from build123d import *

# Parameters (mm, degrees)
SKETCH_1_R      = 1.6
SKETCH_1_R_2    = 1.1
EXTRUDE_1_DEPTH = 5
SKETCH_2_R      = 1.6
SKETCH_2_R_2    = 1.1
EXTRUDE_2_DEPTH = 4
EXTRUDE_START   = 4
SKETCH_3_R      = 1.1
SKETCH_3_R_2    = 1.3
EXTRUDE_3_DEPTH = 4
FILLET_2_R      = 2.5
SKETCH_4_W      = 16
SKETCH_4_H      = 46
EXTRUDE_4_DEPTH = 4
FILLET_3_R      = 5


with BuildPart() as part:
    # Sketch 1 → Extrude 1 (new body)
    with BuildSketch(Plane.XY):
        with BuildLine():
            Line((-8, 0), (8, 0))
            Line((8, 0), (8, 12))
            ThreePointArc((8, 12), (10, 18), (8, 24))
            Line((8, 24), (8, 36))
            Line((8, 36), (-8, 36))
            Line((-8, 36), (-8, 24))
            ThreePointArc((-8, 24), (-10, 18), (-8, 12))
            Line((-8, 12), (-8, 0))
        make_face()
        with Locations((0, 18)):
            Circle(SKETCH_1_R, mode=Mode.SUBTRACT)
        with Locations((0, 24)):
            Circle(SKETCH_1_R_2, mode=Mode.SUBTRACT)
        with Locations((4.242640687, 22.242640687)):
            Circle(SKETCH_1_R_2, mode=Mode.SUBTRACT)
        with Locations((6, 18)):
            Circle(SKETCH_1_R_2, mode=Mode.SUBTRACT)
        with Locations((4.242640687, 13.757359313)):
            Circle(SKETCH_1_R_2, mode=Mode.SUBTRACT)
        with Locations((0, 12)):
            Circle(SKETCH_1_R_2, mode=Mode.SUBTRACT)
        with Locations((-4.242640687, 13.757359313)):
            Circle(SKETCH_1_R_2, mode=Mode.SUBTRACT)
        with Locations((-6, 18)):
            Circle(SKETCH_1_R_2, mode=Mode.SUBTRACT)
        with Locations((-4.242640687, 22.242640687)):
            Circle(SKETCH_1_R_2, mode=Mode.SUBTRACT)
    extrude(amount=EXTRUDE_1_DEPTH)

    # Sketch 2 → Extrude 2 (add)
    with BuildSketch(Plane.XZ):
        with BuildLine():
            Line((-8, 0), (8, 0))
            Line((8, 0), (8, 21))
            ThreePointArc((8, 21), (10, 27), (8, 33))
            Line((8, 33), (8, 37))
            Line((8, 37), (-8, 37))
            Line((-8, 37), (-8, 33))
            ThreePointArc((-8, 33), (-10, 27), (-8, 21))
            Line((-8, 21), (-8, 0))
        make_face()
        with Locations(Location((0, 27, 0), (0, 0, 270))):
            Circle(SKETCH_2_R, mode=Mode.SUBTRACT)
        with Locations(Location((6, 27, 0), (0, 0, 270))):
            Circle(SKETCH_2_R_2, mode=Mode.SUBTRACT)
        with Locations(Location((4.242640687, 22.757359313, 0), (0, 0, 270))):
            Circle(SKETCH_2_R_2, mode=Mode.SUBTRACT)
        with Locations(Location((0, 21, 0), (0, 0, 270))):
            Circle(SKETCH_2_R_2, mode=Mode.SUBTRACT)
        with Locations(Location((-4.242640687, 22.757359313, 0), (0, 0, 270))):
            Circle(SKETCH_2_R_2, mode=Mode.SUBTRACT)
        with Locations(Location((-6, 27, 0), (0, 0, 270))):
            Circle(SKETCH_2_R_2, mode=Mode.SUBTRACT)
        with Locations(Location((-4.242640687, 31.242640687, 0), (0, 0, 270))):
            Circle(SKETCH_2_R_2, mode=Mode.SUBTRACT)
        with Locations(Location((0, 33, 0), (0, 0, 270))):
            Circle(SKETCH_2_R_2, mode=Mode.SUBTRACT)
        with Locations(Location((4.242640687, 31.242640687, 0), (0, 0, 270))):
            Circle(SKETCH_2_R_2, mode=Mode.SUBTRACT)
    extrude(amount=EXTRUDE_2_DEPTH)

    # Sketch 3 → Extrude 3 (add)
    with BuildSketch(Plane(origin=(0, 36, 0), x_dir=(1, 0, 0), z_dir=(0, 1, 0)).offset(EXTRUDE_START)):
        with BuildLine():
            Line((8, -5), (8, 0))
            Line((8, 0), (-8, 0))
            Line((-8, 0), (-8, -5))
            Line((-8, -5), (-8, -21))
            ThreePointArc((-8, -21), (-10, -27), (-8, -33))
            Line((-8, -33), (-8, -37))
            Line((-8, -37), (8, -37))
            Line((8, -37), (8, -33))
            ThreePointArc((8, -33), (10, -27), (8, -21))
            Line((8, -21), (8, -5))
        make_face()
        with Locations(Location((4.242640687, -22.757359313, 0), (0, 0, 90))):
            Circle(SKETCH_3_R, mode=Mode.SUBTRACT)
        with Locations(Location((0, -21, 0), (0, 0, 90))):
            Circle(SKETCH_3_R, mode=Mode.SUBTRACT)
        with Locations(Location((-4.242640687, -22.757359313, 0), (0, 0, 90))):
            Circle(SKETCH_3_R, mode=Mode.SUBTRACT)
        with Locations(Location((-6, -27, 0), (0, 0, 90))):
            Circle(SKETCH_3_R, mode=Mode.SUBTRACT)
        with Locations(Location((-4.242640687, -31.242640687, 0), (0, 0, 90))):
            Circle(SKETCH_3_R, mode=Mode.SUBTRACT)
        with Locations(Location((0, -33, 0), (0, 0, 90))):
            Circle(SKETCH_3_R, mode=Mode.SUBTRACT)
        with Locations(Location((4.242640687, -31.242640687, 0), (0, 0, 90))):
            Circle(SKETCH_3_R, mode=Mode.SUBTRACT)
        with Locations(Location((6, -27, 0), (0, 0, 90))):
            Circle(SKETCH_3_R, mode=Mode.SUBTRACT)
        with Locations(Location((0, -27, 0), (0, 0, 270))):
            Circle(SKETCH_3_R_2, mode=Mode.SUBTRACT)
    extrude(amount=-EXTRUDE_3_DEPTH)

    # Fillet 2
    fillet_2_edges = [part.edges().sort_by_distance(p)[0] for p in [
        (8, 38, 21),
        (-8, 38, 21),
        (-8, 38, 33),
        (-8, 38, 37),
        (8, 38, 37),
        (8, 38, 33),
        (-8, 12, 2.5),
        (-8, 24, 2.5),
        (8, 24, 2.5),
        (8, 12, 2.5),
        (-8, -2, 21),
        (8, -2, 21),
        (8, -2, 33),
        (8, -2, 37),
        (-8, -2, 37),
        (-8, -2, 33),
    ]]
    fillet(fillet_2_edges, radius=FILLET_2_R)


with BuildPart() as body_2:
    # Mirror 2: mirrored copy
    add(part.part.mirror(Plane.XY.offset(-18)))


with BuildPart() as part_1:
    add(part.part)

    add(body_2.part)  # Extrude 4 merges body 2
    # Sketch 4 → Extrude 4 (add)
    with BuildSketch(Plane(origin=(0, 40, 0), x_dir=(1, 0, 0), z_dir=(0, 1, 0))):
        with Locations((0, 18)):
            Rectangle(SKETCH_4_W, SKETCH_4_H)
    extrude(amount=-EXTRUDE_4_DEPTH)

    # Fillet 3
    fillet_3_edges = [part_1.edges().sort_by_distance(p)[0] for p in [
        (0, 36, 5),
        (0, 36, 0),
        (0, 36, -36),
        (0, -4, -36),
        (0, 0, -41),
        (0, 36, -41),
        (0, -4, 0),
        (0, 0, 5),
    ]]
    fillet(fillet_3_edges, radius=FILLET_3_R)


solid = part_1.part
Design review of the part built by this model. Coordinates are the model's own, in mm. A direction names the side the tool comes from. Round coordinates to 2 decimals unless told otherwise and drop trailing zeros. Loops run counter-clockwise (first coordinate to the right, second up) from the corner with the lowest first, then second, coordinate; pieces in that order, holes last. Notation, with made-up numbers: M -26,41 L -21,41 A27 ccw -21,64 Z; hole C -13.5,25 d11. An arc over 180 degrees is marked long. Answer as a JSON object with one key per item and string values.
Item 1: Clearance check with flat-ended pins moving along their axes: P1, Ø6, axis at x = -5, y = 21.5, coming from the -Z side; P2, Ø3.5, axis at x = -6, z = 27, coming from the +Y side; P3, Ø16.5, axis at y = 34.5, z = -32.5, coming from the -X side; P4, Ø3.5, axis at x = 6, y = 18, coming from the +Z side. State where each tip first meets the part, or that it passes through.
Answer sheet:
{"P1": "stops at z = -41", "P2": "stops at y = 40", "P3": "stops at x = -8", "P4": "stops at z = 5"}
Item 2: Machinability: for faces 1 (the flat face through (0, 36, -18)), 2 (the flat face through (0, 0, 24)), 3 (the flat face through (2, 18, -41)), which of the approach directions +Z, -Z, +X, -X, +Y, -Y give a long, thin tool a straight path to every point of the face, cutting with its end or side? Answer none if there is none.
Answer sheet:
{"face 1": "+X, -X, -Y", "face 2": "+Z, +X, -X", "face 3": "-Z, +X, -X"}
Item 3: Wall thickness on L1, parallel to X at y = 38, z = 27; L2, parallel to Y at x = -4.5, z = 18.5; L3, parallel to Z at x = -7, y = 30: over which ranges is each line inside the solid? List them lowest first. Write a range as from..to.
Answer sheet:
{"L1": "x = -10..-7.1, -4.9..-1.3, 1.3..4.9, 7.1..10", "L2": "y = -4..0, 36..40", "L3": "z = -41..-36, 0..5"}
Item 4: We need section A-A on y = 18. State how many separate pieces and enclosed holes the cut face has, and give its area (3 significant figures).
Answer sheet:
{"separate pieces": "8", "enclosed holes": "0", "area": "124 mm^2"}
Item 5: The part is to be moulded in two halves that separate along Y. For faces 4 (the cylindrical face through (0.481, -1.972, -61.474)), 5 (the cylindrical face through (0, -2, -37)), 6 (the cylindrical face through (-0.208, 19.586, 2.465)), say which applies: pulls with the +Y half, pulls with the -Y half, needs draft (parallel to the pull), parting line crosses it, or undercut.
Answer sheet:
{"face 4": "needs draft", "face 5": "pulls with the -Y half", "face 6": "undercut"}
Item 6: We need section C-C on y = 9.5. Give the boundary of the cut face in (x, z).
Answer sheet:
{"outline": "M -8,-41 L 8,-41 L 8,-36 L -8,-36 Z; M -8,0 L 8,0 L 8,5 L -8,5 Z"}
Item 7: We need section D-D on z = 7.5. Give the boundary of the cut face in (x, y), and give its area (3 significant figures).
Answer sheet:
{"outline": "M -8,-4 L 8,-4 L 8,0.67 L -8,0.67 Z; M -8,35.33 L 8,35.33 L 8,40 L -8,40 Z", "area": "149 mm^2"}
